Input: part model. Units: mm. Frame: model coordinates. A direction names the side the tool comes from. Give positions to 0.01 mm unless a question says otherwise; leave off trailing zeros. Order: outer loops, then holes, each group sorted by start corner. A loop starts at its lowest first (then second) coordinate and runs counter-clockwise, first axis right, second up. Notation, with made-up numbers: (-8, 87.25) - (20, 87.25) arc R12 cw to (20, 104.25) - close; hole circle Ø9 at (42, -25). An arc over 180 degrees is marked (long way). Answer in a Markdown table with one row per item. Add a question column.
Autodesk Inventor part; units mm, degrees
ref_plane "YZ Plane" through (0, 0, 0) normal (1, 0, 0) x (0, 1, 0)
ref_plane "XZ Plane" through (0, 0, 0) normal (0, 1, 0) x (-1, 0, 0)
ref_plane "XY Plane" through (0, 0, 0) normal (0, 0, 1) x (1, 0, 0)
sketch "Sketch1" plane through (0, 0, 0) normal (0, 0, 1) x (1, 0, 0)
  line L0 (0, -57.15) -> (0, 57.15) construction
  line L1 (6.35, -57.15) -> (6.35, 57.15)
  line L2 (-6.35, 57.15) -> (-6.35, -57.15)
  arc A0 (-6.35, -57.15) -> (6.35, -57.15) centre (0, -57.15) ccw
  arc A1 (6.35, 57.15) -> (-6.35, 57.15) centre (0, 57.15) ccw
  circle A2 centre (0, 57.15) radius 2.4892
  circle A3 centre (0, -57.15) radius 2.4892
  circle A4 centre (0, 0) radius 5.1562
  circle A5 centre (0, 0) radius 11.1125
  point P0 (-6.35, 9.1195)
  point P1 (-6.35, -9.1195)
  point P2 (6.35, -9.1195)
  point P3 (6.35, 9.1195)
  dimension "d0" = 114.3
  dimension "d1" = 12.7
  dimension "d2" = 4.9784
  dimension "d3" = 10.3124
  dimension "d4" = 22.225
extrude "Extrusion1" add sketch "Sketch1" along normal blind 3.175
sketch "Sketch2" plane through (0, 0, 3.175) normal (0, 0, 1) x (1, 0, 0)
  circle A0 centre (0, 0) radius 15.875 construction
  circle A1 centre (0, 15.875) radius 3.175
  circle A2 centre (0, -15.875) radius 3.175
  dimension "d7" = 31.75
  dimension "d8" = 6.35
  dimension "d9" = 6.35
extrude "Extrusion2" cut sketch "Sketch2" against normal through all
fillet "Fillet1" radius 3.175 4 edges at (6.35, 9.1195, 1.5875) (6.35, -9.1195, 1.5875) (-6.35, -9.1195, 1.5875) (-6.35, 9.1195, 1.5875)
properties part number "EncoderStrip" material "Aluminum 6061"
Q1. Section C-C, the plane z = 2.25. State how many separate pieces and enclosed holes the cut face has, then the cut area to 3 significant figures.
Q2. Access query for faces 1 (the flat face through (-6.35, -34, 2)), 2 (the flat face through (6.35, 34, 2)), 3 (the flat face through (-6.35, 34, 2)), 4 (the cylindrical face through (6.634, -9.336, 1.61)), 5 (the cylindrical face through (-0.32, -59.62, 1.57)). Directions: +Z, -Z, +X, -X, +Y, -Y. A direction counts if a zero-diameter tool reaches every point of the face in a straight line with its end or side. Return the directions, or none.
Q3. Pull-direction query (Y, two-part tool) for faces 6 (the cylindrical face through (2.3, 58.1, 1.6)), 7 (the cylindrical face through (-6.634, 9.336, 1.61)), 8 (the flat face through (6.35, -34, 2)); classes: +Y half, -Y half, draft (parallel to the pull), parting line (faces both ways), or undercut.
Q4. Section A-A, the plane y = 0. Return loops of the section in (x, z) (1 decimal), then the cut area to 3 significant figures.
Q5. Section D-D, the plane y = 40. Return loops of the section in (x, z) (3 decimals).
Q6. Line query: probe 1 along Y at (x, z) = (0, 2.2); probe 2 along Y at (x, z) = (1, 2.35); probe 3 along X at (y, z) = (-36.5, 0.85). Output: solid intervals per line, ascending.
Q7. Section B-B, the plane x = 0. Return loops of the section in (y, z) (3 decimals).
Q8. Contact query for flat-ended pins moving along their axis: P1, Ø4, axis at x = 0, y = -15.875, coming from the -Z side; P2, Ø1, axis at y = 26, z = 1.5, coming from the +X side; P3, Ø1.6, axis at y = -32.5, z = 2, coming from the -X side. Output: stop coordinate, or through.
Computed:
| question | item | result |
|---|---|---|
| 1 | separate pieces | 1 |
| 1 | enclosed holes | 5 |
| 1 | area | 1,520 mm^2 |
| 2 | face 1 | +Z, -Z, -X, -Y |
| 2 | face 2 | +Z, -Z, +X, +Y |
| 2 | face 3 | +Z, -Z, -X, +Y |
| 2 | face 4 | +Z, -Z, +X, -Y |
| 2 | face 5 | +Z, -Z |
| 3 | face 6 | undercut |
| 3 | face 7 | +Y half |
| 3 | face 8 | draft |
| 4 | outline | (-11.1, 0) - (-5.2, 0) - (-5.2, 3.2) - (-11.1, 3.2) - close; (5.2, 0) - (11.1, 0) - (11.1, 3.2) - (5.2, 3.2) - close |
| 4 | area | 37.8 mm^2 |
| 5 | outline | (-6.35, 0) - (6.35, 0) - (6.35, 3.175) - (-6.35, 3.175) - close |
| 6 | probe 1 | y = -63.5 to -59.64, -54.66 to -19.05, -12.7 to -5.16, 5.16 to 12.7, 19.05 to 54.66, 59.64 to 63.5 |
| 6 | probe 2 | y = -63.42 to -59.43, -54.87 to -18.89, -12.86 to -5.06, 5.06 to 12.86, 18.89 to 54.87, 59.43 to 63.42 |
| 6 | probe 3 | x = -6.35 to 6.35 |
| 7 | outline | (-63.5, 0) - (-59.639, 0) - (-59.639, 3.175) - (-63.5, 3.175) - close; (-54.661, 0) - (-19.05, 0) - (-19.05, 3.175) - (-54.661, 3.175) - close; (-12.7, 0) - (-5.156, 0) - (-5.156, 3.175) - (-12.7, 3.175) - close; (5.156, 0) - (12.7, 0) - (12.7, 3.175) - (5.156, 3.175) - close; (19.05, 0) - (54.661, 0) - (54.661, 3.175) - (19.05, 3.175) - close; (59.639, 0) - (63.5, 0) - (63.5, 3.175) - (59.639, 3.175) - close |
| 8 | P1 | passes through |
| 8 | P2 | stops at x = 6.35 |
| 8 | P3 | stops at x = -6.35 |
